```python
from build123d import *

# Parameters (mm, degrees)
SKETCH_1_W          = 64
SKETCH_1_H          = 48.5
EXTRUDE_1_DEPTH     = 3
EXTRUDE_2_DEPTH     = 50
FILLET_2_R          = 2
SKETCH_3_R          = 2
CUT_EXTRUDE_1_DEPTH = 65
FILLET_3_R          = 2


with BuildPart() as part:
    # Эскиз1 → Бобышка-Вытянуть1 (new body)
    with BuildSketch(Plane(origin=(0, 0, 0), x_dir=(1, 0, 0), z_dir=(0, 1, 0))):
        Rectangle(SKETCH_1_W, SKETCH_1_H)
    extrude(amount=EXTRUDE_1_DEPTH)

    # Эскиз2 → Бобышка-Вытянуть2 (add)
    with BuildSketch(Plane(origin=(0, 3, 0), x_dir=(1, 0, 0), z_dir=(0, 1, 0))):
        Polygon((-32, -24.25), (-32, 24.25), (32, 24.25), (32, -24.25), (29, -24.25), (29, 21.25), (-29, 21.25), (-29, -24.25), align=None)
    extrude(amount=EXTRUDE_2_DEPTH)

    # Скругление2
    fillet_2_edges = [part.edges().sort_by_distance(p)[0] for p in [
        (0, 0, -24.25),
    ]]
    fillet(fillet_2_edges, radius=FILLET_2_R)

    # Эскиз3 → Вырез-Вытянуть1 (cut, through all)
    with BuildSketch(Plane(origin=(32, 0, 0), x_dir=(0, 0, -1), z_dir=(1, 0, 0))):
        with Locations((8.75, 28)):
            Circle(SKETCH_3_R)
        with Locations((-3.75, 28)):
            Circle(SKETCH_3_R)
        with Locations((-16.25, 28)):
            Circle(SKETCH_3_R)
    extrude(amount=-CUT_EXTRUDE_1_DEPTH, mode=Mode.SUBTRACT)

    # Скругление3
    fillet_3_edges = [part.edges().sort_by_distance(p)[0] for p in [
        (-29, 3, 1.5),
        (-29, 28, -21.25),
        (29, 3, 1.5),
        (29, 28, -21.25),
        (-32, 0, 1),
        (-32, 0.585786438, -23.664213562),
        (32, 0.585786438, -23.664213562),
        (32, 0, 1),
        (-32, 27.5, -24.25),
        (32, 27.5, -24.25),
    ]]
    fillet(fillet_3_edges, radius=FILLET_3_R)


solid = part.part
```
Could you check a few things on this model? Use its own coordinates, in mm. A direction names the side the tool comes from. Round coordinates to 2 decimals unless told otherwise and drop trailing zeros. Loops run counter-clockwise (first coordinate to the right, second up) from the corner with the lowest first, then second, coordinate; pieces in that order, holes last.
Q1. I want a section at D-D (z = 11.5). Write out the boundary of the cut face in (x, y), and give its area (3 significant figures).
Q2. Please list where these lines run through material, in increasing order: L1, parallel to X at y = 9, z = -13; L2, parallel to Z at x = -15.5, y = 42; L3, parallel to Y at x = 7, z = 5.
Q3. I want a section at A-A (z = 3.75). Write out the boundary of the cut face in (x, y).
Q4. On a 3-axis mill with a long thin cutter (end or side, diameter ignored), from which of +Z, -Z, +X, -X, +Y, -Y can I reach the whole of each face in a straight line? I mean faces 1 (the cylindrical face through (0.42, 0.57, -23.65)), 2 (the flat face through (29, 29, -2)). Say none if no direction works.
Q5. Thinking about a two-plate mould opening in X: for faces 3 (the cylindrical face through (-31.43, 27.86, -23.65)), 4 (the flat face through (0, 27, -24.25)), 5 (the cylindrical face through (28.43, 3.6, 1.18)), 6 (the cylindrical face through (31.4, 27.86, -23.68)), which applies, pulls with the +X half, pulls with the -X half, needs draft (parallel to the pull), parting line crosses it, or undercut?
Q6. For P1, Ø8, axis at x = -9, y = 30, coming from the +Z side; P2, Ø8, axis at x = -8, z = -2, coming from the +Y side, each with a flat end and sliding along its axis, tell me the tip position at first contact or that it passes through.
Q7. I want a section at B-B (x = 10). Write out the boundary of the cut face in (y, z), and give its area (3 significant figures).
Q8. I want a section at C-C (y = 12). Write out the boundary of the cut face in (x, z), and give its area (3 significant figures).
Answer below:
1. outline: (-32, 2) arc R2 ccw to (-30, 0) - (30, 0) arc R2 ccw to (32, 2) - (32, 53) - (29, 53) - (29, 5) arc R2 cw to (27, 3) - (-27, 3) arc R2 cw to (-29, 5) - (-29, 53) - (-32, 53) - close
1. area: 492 mm2
2. L1: x = -32 to -29, 29 to 32
2. L2: z = -24.25 to -21.25
2. L3: y = 0 to 3
3. outline: (-32, 2) arc R2 ccw to (-30, 0) - (30, 0) arc R2 ccw to (32, 2) - (32, 26) - (29, 26) - (29, 5) arc R2 cw to (27, 3) - (-27, 3) arc R2 cw to (-29, 5) - (-29, 26) - (-32, 26) - close; (-32, 30) - (-29, 30) - (-29, 53) - (-32, 53) - close; (29, 30) - (32, 30) - (32, 53) - (29, 53) - close
4. face 1: -Z, +X, -X, -Y
4. face 2: +Z, +Y
5. face 3: pulls with the -X half
5. face 4: needs draft
5. face 5: undercut
5. face 6: pulls with the +X half
6. P1: stops at z = -21.25
6. P2: stops at y = 3
7. outline: (0, -22.25) arc R2 ccw to (2, -24.25) - (53, -24.25) - (53, -21.25) - (3, -21.25) - (3, 24.25) - (0, 24.25) - close
7. area: 295 mm2
8. outline: (-32, -22.25) arc R2 ccw to (-30, -24.25) - (30, -24.25) arc R2 ccw to (32, -22.25) - (32, 24.25) - (29, 24.25) - (29, -19.25) arc R2 cw to (27, -21.25) - (-27, -21.25) arc R2 cw to (-29, -19.25) - (-29, 24.25) - (-32, 24.25) - close
8. area: 465 mm2
